Geometry: final body of the model. Coordinates: model frame, mm. Face numbers are marked on the shaded views. Give positions to 0.01 mm unless a question says otherwise; leave off trailing zeros. Write each loop counter-clockwise with the first axis right and the second up, starting at its lowest first coordinate (ties: lowest second). Pieces come first, ordered by that corner, then holes.
```python
from build123d import *

# Parameters (mm, degrees)
SKETCH1_R           = 10
BOSS_EXTRUDE1_DEPTH = 13


with BuildPart() as part:
    # Sketch1 → Boss-Extrude1 (new body)
    with BuildSketch(Plane(origin=(0, 0, 0), x_dir=(0, 0, -1), z_dir=(1, 0, 0))):
        Polygon((-16, 9.237604307), (-16, -9.237604307), (0, -18.475208614), (16, -9.237604307), (16, 9.237604307), (0, 18.475208614), align=None)
        with Locations(Location((0, 0, 0), (0, 0, 180))):
            Circle(SKETCH1_R, mode=Mode.SUBTRACT)
    extrude(amount=BOSS_EXTRUDE1_DEPTH)

    # Sketch2 → Cut-Revolve1 (revolve, cut)
    with BuildSketch(Plane(origin=(0, 0, 0), x_dir=(1, 0, 0), z_dir=(0, 1, 0)), mode=Mode.PRIVATE) as cut_revolve1_sk:
        Polygon((0, 14.5), (3.137550133, 19.521191174), (-1.152758785, 19.521191174), (-1.152758785, 14.5), align=None)
    revolve(cut_revolve1_sk.sketch.rotate(Axis((0, 0, 0), (1, 0, 0)), 29.999999997), axis=Axis((0, 0, 0), (1, 0, 0)), mode=Mode.SUBTRACT)

    # Sketch4 → Revolve1 (revolve)
    with BuildSketch(Plane(origin=(0, 0, 0), x_dir=(1, 0, 0), z_dir=(0, 1, 0)), mode=Mode.PRIVATE) as revolve1_sk:
        with BuildLine():
            Line((0, 11.75), (0, 14.5))
            ThreePointArc((0, 14.5), (-1.375, 13.125), (0, 11.75))
        make_face()
    revolve(revolve1_sk.sketch.rotate(Axis((0, 0, 0), (1, 0, 0)), 180), axis=Axis((0, 0, 0), (1, 0, 0)))


solid = part.part
```
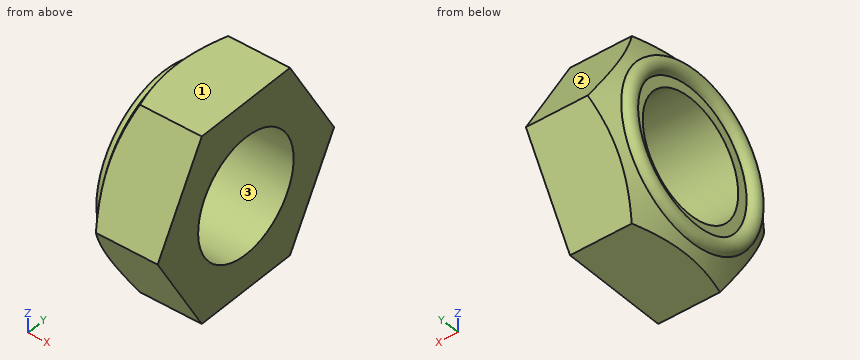
Item 1: Pull-direction query (Y, two-part tool) for the marked faces 1, 2 and 3; classes: +Y half, -Y half, draft (parallel to the pull), parting line (faces both ways), or undercut.
Found:
face 1: draft
face 2: +Y half
face 3: undercut
Item 2: Section B-B, the plane y = 0. Return the cut outline in (x, z) (3 decimals).
Found:
outline: (0, -14.5) - (0.937, -16) - (13, -16) - (13, -10) - (0, -10) - (0, -11.75) arc R1.375 ccw to start; (0, 10) - (13, 10) - (13, 16) - (0.937, 16) - (0, 14.5) arc R1.375 ccw to (0, 11.75) - close
Item 3: Section A-A, the plane x = 3.5. Return the cut outline in (y, z), plus the area to 3 significant figures.
Found:
outline: (-18.48, 0) - (-9.24, -16) - (9.24, -16) - (18.48, 0) - (9.24, 16) - (-9.24, 16) - close; hole circle Ø20 at (0, 0)
area: 573 mm2
Item 4: Line query: L1, parallel to Y at x = 8.75, z = 0; L2, parallel to X at y = 15.5, z = 4; L3, parallel to Y at x = 6.5, z = 8.5. Output: solid intervals per line, ascending.
Found:
L1: y = -18.48 to -10, 10 to 18.48
L2: x = 0.94 to 13
L3: y = -13.57 to -5.27, 5.27 to 13.57
Item 5: Pin query (flat end, axial travel): pin 1 Ø19 at (y, z) = (-1.5, 1.5) entering from -X; pin 2 Ø16 at (y, z) = (0, 0) entering from -X; pin 3 Ø1 at (x, z) = (4, -13) entering from -Y; pin 4 Ø1 at (x, y) = (6.5, 10.5) entering from -Z. Return the tip coordinate at first contact, or that it passes through.
Found:
pin 1: stops at x = 0
pin 2: passes through
pin 3: stops at y = -11.26
pin 4: stops at z = -14.68
